Source: three-view drawing plus pictorial views. Frame: mm from the lowest corner of the part. Round coordinates to 2 decimals unless told otherwise and drop trailing zeros. Loops run counter-clockwise (first coordinate to the right, second up) from the corner with the lowest first, then second, coordinate; pieces in that order, holes last. Notation, with made-up numbers: (0.5, -6) -> (23.5, -6) arc R16 ccw to (23.5, 3) -> close; hole circle Ø8 at (-9.5, 67). An arc over 180 degrees is marked (long way). Answer in a Markdown table with one row per item.
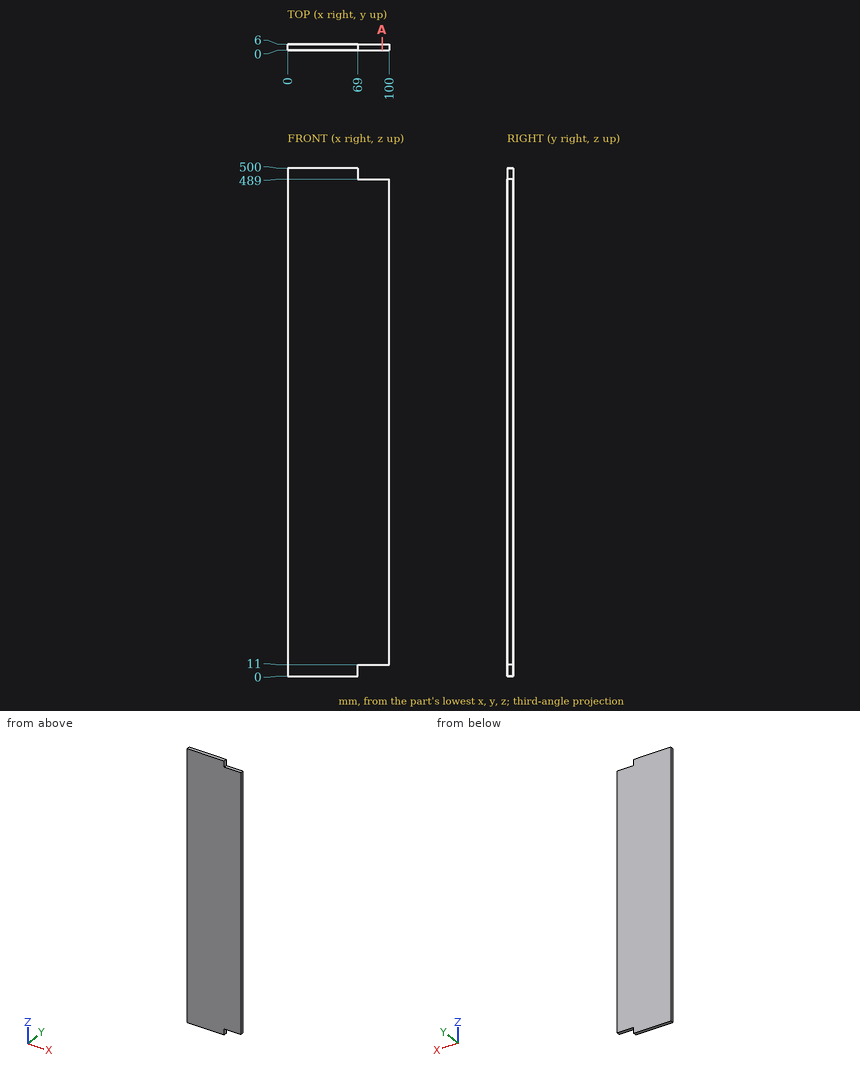
Item 1: Line query: probe 1 along Z at (x, y) = (74.5, 3.8). Output: solid intervals per line, ascending. Write a range as [from, to].
Answer:
| item | result |
|---|---|
| probe 1 | z = [11, 489] |
Item 2: Cut plane A-A (x = 93). Output: boundary loops of the cut face in (y, z), then the cut area to 3 significant figures.
Answer:
| item | result |
|---|---|
| outline | (0, 11) -> (6, 11) -> (6, 489) -> (0, 489) -> close |
| area | 2,870 mm² |
Item 3: Pin query (flat end, axial travel): pin 1 Ø3 at (x, y) = (81, 4.5) entering from -Z; pin 2 Ø3 at (x, y) = (82, 4) entering from +Z; pin 3 Ø1.8 at (y, z) = (4, 492) entering from +X. Return the tip coordinate at first contact, or that it passes through.
Answer:
| item | result |
|---|---|
| pin 1 | stops at z = 11 |
| pin 2 | stops at z = 489 |
| pin 3 | stops at x = 69 |
